Geometry: final body of the model. Coordinates: model frame, mm. A direction names the side the tool comes from. Give positions to 0.01 mm unless a question says otherwise; leave off trailing zeros. Write each loop counter-clockwise with the first axis right and the second up, starting at its lowest first coordinate (ties: lowest second). Pieces come first, ordered by that corner, then holes.
Q1. Pin query (flat end, axial travel): pin 1 (1.5 mm diameter, centred on y = 1.5, z = 17, fed in from +X); pin 2 (12 mm diameter, centred on x = 10, z = 6, fed in from -Y). Return the tip coordinate at first contact, or that it passes through.
Q2. Cut plane C-C on z = 5.5. Return the cut outline in (x, y).
Q3. Cut plane B-B on y = 5.5. Return the cut outline in (x, z), plus the area to 3 significant figures.
Q4. Cut plane D-D on x = 16. Return the cut outline in (y, z).
Q5. Draft query along Y for faces 1 (the face through (-0.74, 3.65, 7.66)), 2 (the face through (5.3, 10, 20.3)), 3 (the face through (-0.83, 4.93, 20.86)), 4 (the face through (-0.739, 4.627, 17.886)). Return one class per face: pulls with the +Y half, pulls with the -Y half, needs draft (parallel to the pull), parting line crosses it, or undercut.
Q6. Reachability of faces 5 (the face through (20, 5, 21)), 6 (the face through (10, 5, 20)) from +Z, -Z, +X, -X, +Y, -Y: full face, straight path, thin tool, end or side. Return the list, or none.
Q7. Line query: L1, parallel to Z at x = 6.25, y = 5.5; L2, parallel to X at y = 7.5, z = 10.75. Output: solid intervals per line, ascending.
Q8. Cut plane A-A on y = 9. Return the cut outline in (x, z).
```python
from build123d import *

# Parameters (mm, degrees)
BASE_FLANGE1_DEPTH                 = 10
F_3_0MM_TRANSITIONAL_DOWEL_HOLE1_D = 3


# Sheet-metal steps are written as plain solids
with BuildPart() as part:
    # Sketch1 → Base-Flange1 (new body)
    with BuildSketch(Plane(origin=(0, 0, 0), x_dir=(1, 0, 0), z_dir=(0, 1, 0))):
        with BuildLine():
            Line((0, 0), (0, -19.2634))
            ThreePointArc((0, -19.2634), (0.215745145, -19.784254855), (0.7366, -20))
            Line((0.7366, -20), (20, -20))
            Line((20, -20), (20, -21.5))
            Line((20, -21.5), (0.7366, -21.5))
            ThreePointArc((0.7366, -21.5), (-0.844915027, -20.844915027), (-1.5, -19.2634))
            Line((-1.5, -19.2634), (-1.5, 0))
            Line((-1.5, 0), (0, 0))
        make_face()
    extrude(amount=BASE_FLANGE1_DEPTH)

    # Ø3.0mm Transitional Dowel Hole1 (through all)
    with Locations(Plane.ZY.offset(1.5)):
        with Locations((16.387023366, 4.560762846), (6.466703516, 4.560762846)):
            Hole(F_3_0MM_TRANSITIONAL_DOWEL_HOLE1_D / 2)


solid = part.part
```
Data:
1. pin 1: stops at x = 0
1. pin 2: passes through
2. outline: (-1.5, 0) - (0, 0) - (0, 3.41) - (-1.5, 3.41) - close; (-1.5, 5.71) - (0, 5.71) - (0, 10) - (-1.5, 10) - close
3. outline: (-1.5, 0) - (0, 0) - (0, 5.3) - (-1.5, 5.3) - close; (-1.5, 7.64) - (0, 7.64) - (0, 15.22) - (-1.5, 15.22) - close; (-1.5, 17.56) - (0, 17.56) - (0, 19.26) arc R0.74 cw to (0.74, 20) - (20, 20) - (20, 21.5) - (0.74, 21.5) arc R2.24 ccw to (-1.5, 19.26) - close
3. area: 54.3 mm2
4. outline: (0, 20) - (10, 20) - (10, 21.5) - (0, 21.5) - close
5. face 1: undercut
5. face 2: pulls with the +Y half
5. face 3: needs draft
5. face 4: undercut
6. face 5: +Z, -Z, +X, +Y, -Y
6. face 6: -Z, +X, +Y, -Y
7. L1: z = 20 to 21.5
7. L2: x = -1.5 to 0
8. outline: (-1.5, 0) - (0, 0) - (0, 19.26) arc R0.74 cw to (0.74, 20) - (20, 20) - (20, 21.5) - (0.74, 21.5) arc R2.24 ccw to (-1.5, 19.26) - close
